Geometry: final body of the model. Coordinates: model frame, mm. Face numbers are marked on the shaded views. A direction names the side the tool comes from. Give positions to 0.01 mm unless a question says otherwise; leave off trailing zeros. Write each loop counter-clockwise with the first axis right and the second up, starting at its lowest first coordinate (ties: lowest second). Pieces come first, ordered by that corner, then holes. Notation, with made-up numbers: M -2,38 L 14,38 A3 cw 14,43 Z; hole C 27.25,64 d9. An arc over 180 degrees is marked long. Use a Markdown table: item, result. Add a question column.
1) Set-up query: the marked faces 1 and 2. Return all of +Z, -Z, +X, -X, +Y, -Y with unobstructed straight access to the full face (end or side cutting, diameter ignored); none if empty.
2) Section A-A on x = -7. Return the cut outline in (y, z), then the cut area to 3 significant figures.
3) Section B-B on y = -9. Return the cut outline in (x, z).
4) Line query: line 1 (Y direction, x = 1, z = 0.5); line 2 (Z direction, x = -15, y = -7); line 3 (Y direction, x = 3, z = 9). Output: solid intervals per line, ascending.
5) Section D-D on z = 6. Return the cut outline in (x, y), then the cut area to 3 significant figures.
6) Section C-C on x = 14.5. Return the cut outline in (y, z), then the cut area to 3 significant figures.
7) Pin query (flat end, axial travel): pin 1 (1 mm diameter, centred on x = 12, z = 2.5, fed in from -Y); pin 2 (0.8 mm diameter, centred on y = -13.5, z = 0.5, fed in from -X); pin 3 (11.5 mm diameter, centred on x = -7.5, y = -19, fed in from +Z). Return the tip coordinate at first contact, or that it passes through.
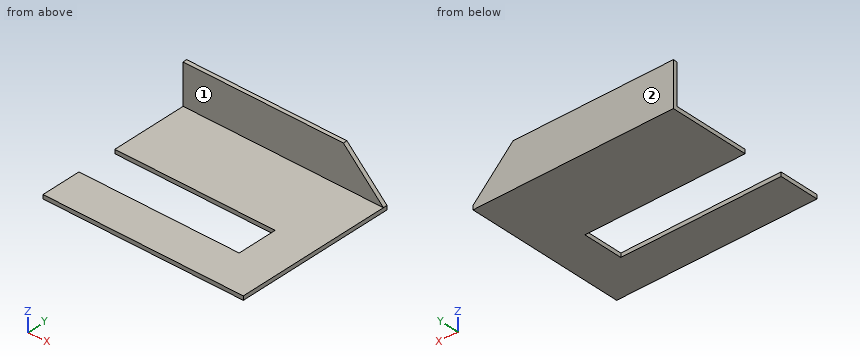
```python
from build123d import *

# Parameters (mm, degrees)
EXTRUDE_1_DEPTH = 1
SKETCH_2_W      = 50
SKETCH_2_H      = 1
EXTRUDE_2_DEPTH = 10
CHAMFER_1_SIZE  = 10


with BuildPart() as part:
    # 草图1 → 凸台-拉伸1 (new body)
    with BuildSketch(Plane.XY):
        Polygon((23.496790028, -8.332562617), (23.496790028, -17.864815409), (23.496790028, -30.601283989), (-26.503209972, -30.601283989), (-26.503209972, -20.601283989), (13.496790028, -20.601283989), (13.496790028, -10.601283989), (-26.503209972, -10.601283989), (-26.503209972, 9.398716011), (23.496790028, 9.398716011), align=None)
    extrude(amount=EXTRUDE_1_DEPTH)

    # 草图2 → 凸台-拉伸2 (add)
    with BuildSketch(Plane.XY.offset(1)):
        with Locations((-1.503209972, 8.898716011)):
            Rectangle(SKETCH_2_W, SKETCH_2_H)
    extrude(amount=EXTRUDE_2_DEPTH)

    # 倒角1
    chamfer_1_edges = [part.edges().sort_by_distance(p)[0] for p in [
        (23.496790028, 8.898716011, 11),
    ]]
    chamfer(chamfer_1_edges, length=CHAMFER_1_SIZE)


solid = part.part
```
Found:
| question | item | result |
|---|---|---|
| 1 | face 1 | +Z, +X, -X, -Y |
| 1 | face 2 | +Z, -Z, +X, -X, +Y |
| 2 | outline | M -30.6,0 L -20.6,0 L -20.6,1 L -30.6,1 Z; M -10.6,0 L 9.4,0 L 9.4,11 L 8.4,11 L 8.4,1 L -10.6,1 Z |
| 2 | area | 40.0 mm² |
| 3 | outline | M -26.5,0 L 23.5,0 L 23.5,1 L -26.5,1 Z |
| 4 | line 1 | -30.6 to -20.6, -10.6 to 9.4 |
| 4 | line 2 | 0 to 1 |
| 4 | line 3 | 8.4 to 9.4 |
| 5 | outline | M -26.5,8.4 L 18.5,8.4 L 18.5,9.4 L -26.5,9.4 Z |
| 5 | area | 45.0 mm² |
| 6 | outline | M -30.6,0 L 9.4,0 L 9.4,10 L 8.4,10 L 8.4,1 L -30.6,1 Z |
| 6 | area | 49.0 mm² |
| 7 | pin 1 | y = 8.4 |
| 7 | pin 2 | x = 13.5 |
| 7 | pin 3 | z = 1 |
